Design review of the part shown in the three views and the two pictorial views. Dimensions are in mm from the part's minimum x, y and z. Coordinates: 2 decimals unless noted, no trailing zeros. Order: outer loops, then holes, each group sorted by start corner. A loop starts at its lowest first (then second) coordinate and runs counter-clockwise, first axis right, second up. Notation, with made-up numbers: (80.5, 9) -> (139.5, 9) arc R17 ccw to (139.5, 21) -> close; hole circle Ø3 at (30.25, 85.25). An arc over 180 degrees is marked (long way). Write item = value, one per line. Start each with the question number.
1) Insertion check: pin 1 Ø1.2 at (x, z) = (2, 3.5) entering from -Y; pin 2 Ø1.5 at (x, y) = (1.5, 9.5) entering from +Z. Each pin has a flat end and moves straight along its axis. Give the tip position at first contact, or say it passes through.
2) Consider section A-A on y = 31. Give the boundary of the cut face in (x, z).
3) Wall thickness on probe 1 along Z at (x, y) = (1, 31); probe 2 along Z at (x, y) = (2.6, 8); probe 3 along Z at (x, y) = (2.4, 41): over which ranges is each line inside the solid? List them lowest first. Write a range as [from, to].
4) Consider section C-C on y = 19. Give the boundary of the cut face in (x, z).
5) Consider section B-B on x = 2.1. Give the boundary of the cut face in (y, z), and give its area (3 significant figures).
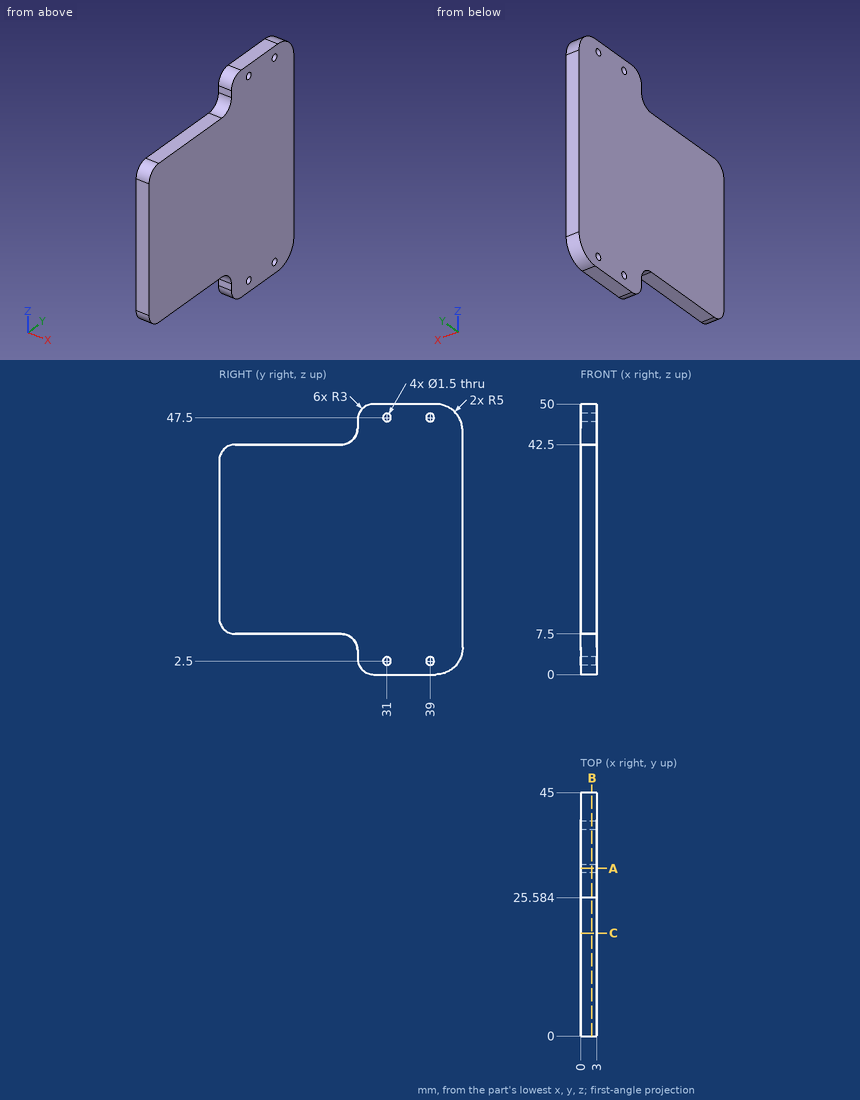
Answer sheet:
q1.pin_1 = 25.58
q1.pin_2 = 42.5
q2.outline = (0, 0) -> (3, 0) -> (3, 1.75) -> (0, 1.75) -> close; (0, 3.25) -> (3, 3.25) -> (3, 46.75) -> (0, 46.75) -> close; (0, 48.25) -> (3, 48.25) -> (3, 50) -> (0, 50) -> close
q3.probe_1 = [0, 1.75], [3.25, 46.75], [48.25, 50]
q3.probe_2 = [7.5, 42.5]
q3.probe_3 = [0.1, 49.9]
q4.outline = (0, 7.5) -> (3, 7.5) -> (3, 42.5) -> (0, 42.5) -> close
q5.outline = (0, 10.5) arc R3 ccw to (3, 7.5) -> (22.58, 7.5) arc R3 cw to (25.58, 4.5) -> (25.58, 3) arc R3 ccw to (28.58, 0) -> (40, 0) arc R5 ccw to (45, 5) -> (45, 45) arc R5 ccw to (40, 50) -> (28.58, 50) arc R3 ccw to (25.58, 47) -> (25.58, 45.5) arc R3 cw to (22.58, 42.5) -> (3, 42.5) arc R3 ccw to (0, 39.5) -> close; hole circle Ø1.5 at (31, 2.5); hole circle Ø1.5 at (31, 47.5); hole circle Ø1.5 at (39, 2.5); hole circle Ø1.5 at (39, 47.5)
q5.area = 1,840 mm2
